The model under review builds one solid part; all positions refer to its coordinate system, in mm. A direction names the side the tool comes from. Round coordinates to 2 decimals unless told otherwise and drop trailing zeros. Write each loop counter-clockwise with the first axis right and the second up, starting at its lowest first coordinate (ties: lowest second). Pieces come first, ordered by that corner, then holes. Notation, with made-up numbers: M 12,-21.75 L 70,-21.75 A16 ccw 70,7.25 Z; hole C 75.25,42 d4. An arc over 180 degrees is marked long. One line per item, written item: value. Start each with the question number.
1) Tool access review of faces 4 (the face through (22.022, -18.882, 1.565)), 5 (the face through (-3, -12, 0)), 6 (the face through (-7.22, -8, 2)), 7 (the face through (2.78, -8, 2)), 8 (the face through (27.72, -17.74, 1.57)): name each direction out of +Z, -Z, +X, -X, +Y, -Y from which nothing blocks a thin tool from reaching the whole face with its end or side.
2) For P1, Ø1, axis at x = 15.5, z = 1.5, coming from the +Y side; P2, Ø3, axis at x = -5.5, y = -16.5, coming from the +Z side; P3, Ø1, axis at y = -8, z = 2, coming from the -X side; P4, Ø8, axis at x = 5.5, y = -21, coming from the -Z side, all flat-tipped, find the tip position at first contact; note any pin that passes through.
3) Mouldability with a two-part tool opening along X and no side actions: class faces 1 (the face through (-2, -6.185, 2)), 2 (the face through (-2, -24.226, 2)), 3 (the face through (23.01, -28.33, 1.57)) as +X half, -X half, draft (parallel to the pull), parting line (faces both ways), or undercut.
4) Wall thickness on probe 1 along Y at (x, z) = (-9, 0.85); probe 2 along Y at (x, z) = (-1.5, 1.8); probe 3 along X at (y, z) = (-9, 1.55): over which ranges is each line inside the solid? List them lowest first.
5) Take a section at D-D, the plane y = -27. Write out the cut boundary in (x, z) (3 decimals), and give its area (3 significant figures).
6) Take a section at B-B, the plane z = 2. Write out the cut boundary in (x, y), and give its area (3 significant figures).
7) Take a section at C-C, the plane y = -21.5. Write out the cut boundary in (x, z) (3 decimals).
8) Take a section at A-A, the plane x = 0.5. Write out the cut boundary in (y, z) (3 decimals).
from build123d import *

# Parameters (mm, degrees)
F1_DEPTH = 3.175


with BuildPart() as f1:
    # F0 (on Top) → F1 (new body)
    with BuildSketch(Plane.XY):
        with BuildLine():
            Line((-7.220087, -9.359666), (-35.094466, -9.359666))
            Line((-35.094466, -9.359666), (-29.309166, -25.879119))
            ThreePointArc((-29.309166, -25.879119), (-27.483004, -28.304664), (-24.590185, -29.226478))
            Line((-24.590185, -29.226478), (20.150011, -29.226478))
            ThreePointArc((20.150011, -29.226478), (23.04283, -28.304664), (24.868992, -25.879119))
            Line((24.868992, -25.879119), (30.654292, -9.359666))
            Line((30.654292, -9.359666), (2.779913, -9.359666))
            Line((2.779913, -9.359666), (2.779913, -6.184666))
            Line((2.779913, -6.184666), (-2.220087, -6.184666))
            Line((-2.220087, -6.184666), (-7.220087, -6.184666))
            Line((-7.220087, -6.184666), (-7.220087, -9.359666))
        make_face()
        with BuildLine():
            Line((-7.220087, -14.359667), (2.779913, -14.359667))
            Line((2.779913, -14.359667), (20.870817, -14.359667))
            ThreePointArc((20.870817, -14.359667), (22.452994, -15.177171), (22.701597, -16.940632))
            Line((22.701597, -16.940632), (21.322294, -20.879118))
            ThreePointArc((21.322294, -20.879118), (19.496132, -23.304663), (16.603314, -24.226477))
            Line((16.603314, -24.226477), (-21.043488, -24.226477))
            ThreePointArc((-21.043488, -24.226477), (-23.936306, -23.304663), (-25.762468, -20.879118))
            Line((-25.762468, -20.879118), (-27.141771, -16.940632))
            ThreePointArc((-27.141771, -16.940632), (-26.893168, -15.177171), (-25.310991, -14.359667))
            Line((-25.310991, -14.359667), (-7.220087, -14.359667))
        make_face(mode=Mode.SUBTRACT)
    extrude(amount=F1_DEPTH)


solid = f1.part
Checked values:
1. face 4: +Z, -Z
1. face 5: -Z, +X, -X, +Y, -Y
1. face 6: +Z, -Z, -X, +Y
1. face 7: +Z, -Z, +X, +Y
1. face 8: +Z, -Z, +X, -Y
2. P1: stops at y = -9.36
2. P2: passes through
2. P3: stops at x = -7.22
2. P4: stops at z = 0
3. face 1: draft
3. face 2: undercut
3. face 3: +X half
4. probe 1: y = -29.23 to -24.23, -14.36 to -9.36
4. probe 2: y = -29.23 to -24.23, -14.36 to -6.18
4. probe 3: x = -7.22 to 2.78
5. outline: M -28.75,0 L 24.31,0 L 24.31,3.175 L -28.75,3.175 Z
5. area: 168 mm2
6. outline: M -35.09,-9.36 L -29.31,-25.88 A5 ccw -24.59,-29.23 L 20.15,-29.23 A5 ccw 24.87,-25.88 L 30.65,-9.36 L 2.78,-9.36 L 2.78,-6.18 L -7.22,-6.18 L -7.22,-9.36 Z; hole M -27.14,-16.94 L -25.76,-20.88 A5 ccw -21.04,-24.23 L 16.6,-24.23 A5 ccw 21.32,-20.88 L 22.7,-16.94 A1.94 ccw 20.87,-14.36 L -25.31,-14.36 A1.94 ccw Z
6. area: 728 mm2
7. outline: M -30.843,0 L -25.497,0 L -25.497,3.175 L -30.843,3.175 Z; M 21.057,0 L 26.403,0 L 26.403,3.175 L 21.057,3.175 Z
8. outline: M -29.226,0 L -24.226,0 L -24.226,3.175 L -29.226,3.175 Z; M -14.36,0 L -6.185,0 L -6.185,3.175 L -14.36,3.175 Z
